Input: part model. Units: mm. Frame: model coordinates. A direction names the side the tool comes from. Round coordinates to 2 decimals unless told otherwise and drop trailing zeros. Order: outer loops, then holes, each group sorted by start corner. A loop starts at its lowest first (then second) coordinate and runs counter-clockwise, first axis right, second up.
Item 1: Cut plane D-D on y = 64. Output: boundary loops of the cut face in (x, z).
Item 2: Reachability of faces 5 (the flat face through (-58, 21, 0)), 6 (the flat face through (-58, 74, 73)), 7 (the flat face through (-58, 67, 58.25)) from +Z, -Z, +X, -X, +Y, -Y: full face, straight path, thin tool, end or side. Return the list, or none.
Item 3: Line query: L1, parallel to Z at x = -57.4, y = 67.25; L2, parallel to Z at x = -57.95, y = -17; L3, parallel to Z at x = -56.8, y = 68.5. Output: solid intervals per line, ascending.
Item 4: Cut plane A-A on y = 13.5. Output: boundary loops of the cut face in (x, z).
Item 5: Mould query, pull axis Y, two halves, no side actions, for faces 1 (the flat face through (-58, -33.5, 5)), 2 (the flat face through (-58, -38.5, 37)), 3 (the flat face through (-58, 22, 6)), 4 (the flat face through (-56.5, 21, 37)). Classes: released by +Y, released by -Y, zero draft, split by the parting line, or undercut.
Item 6: Cut plane B-B on z = 66. Output: boundary loops of the cut face in (x, y).
Item 7: Cut plane C-C on x = -58.75. Output: boundary loops of the cut face in (y, z), then the cut area to 3 significant figures.
Item 8: First-contact query: pin 1 (1.5 mm diameter, centred on x = -58.5, y = 72.5, fed in from +Z). Flat tip, straight axial feed; report the tip coordinate or a pass-through.
Autodesk Inventor part; units mm, degrees
ref_plane "YZ Plane" through (0, 0, 0) normal (1, 0, 0) x (0, 1, 0)
ref_plane "XZ Plane" through (0, 0, 0) normal (0, 1, 0) x (-1, 0, 0)
ref_plane "XY Plane" through (0, 0, 0) normal (0, 0, 1) x (1, 0, 0)
sketch "Sketch1" plane through (0, 0, 0) normal (0, 0, 1) x (1, 0, 0)
  line L0 (-56.5, -25) -> (-59.5, -25)
  line L1 (-59.5, -25) -> (-59.5, 65)
  line L2 (-56.5, -38) -> (-56.5, 78)
  line L3 (-59.5, 65) -> (-56.5, 65)
  line L4 (-56.5, -25) -> (-59.5, -25)
  line L5 (-59.5, -25) -> (-59.5, 65)
  line L6 (-59.5, 65) -> (-56.5, 65)
  line L7 (-56.5, 65) -> (-56.5, -25)
  point P0 (0, 0)
extrude "Extrusion1" add sketch "Sketch1" along normal blind 76
sketch "Sketch2" plane through (-59.5, -25, 0) normal (0, -1, 0) x (1, 0, 0)
  line L0 (3, 0) -> (3, 76)
  line L1 (0, 76) -> (3, 76)
  line L2 (3, 0) -> (0, 0)
  line L3 (0, 0) -> (0, 76)
  line L4 (0, 76) -> (3, 76)
  line L5 (3, 76) -> (3, 0)
  point P0 (59.5, 0)
extrude "Extrusion2" add sketch "Sketch2" along normal blind 13.5
sketch "Sketch4" plane through (-59.5, 65, 0) normal (0, 1, 0) x (1, 0, 0)
  line L0 (3, 0) -> (3, -76)
  line L1 (3, 0) -> (0, 0)
  line L2 (3, -76) -> (0, -76)
  line L3 (0, -76) -> (0, 0)
  line L4 (0, 0) -> (3, 0)
  line L5 (3, 0) -> (3, -76)
  point P0 (59.5, 0)
extrude "Extrusion3" add sketch "Sketch4" along normal blind 16.5
sketch "Sketch5" plane through (-59.5, -38.5, 0) normal (-1, 0, 0) x (0, 0, 1)
  line L0 (0, 120) -> (76, 120)
  line L1 (76, 120) -> (73, 120)
  line L2 (73, 120) -> (73, 110)
  line L3 (73, 110) -> (76, 110)
  line L4 (76, 110) -> (76, 120)
  line L5 (76, 0) -> (76, 120)
  line L6 (76, 0) -> (73, 0)
  line L7 (73, 0) -> (73, 10)
  line L8 (73, 10) -> (76, 10)
  line L9 (76, 10) -> (76, 0)
  point P0 (0, 38.5)
  dimension "d10" = 3
  dimension "d11" = 10
  dimension "d12" = 3
  dimension "d13" = 10
extrude "Extrusion4" cut sketch "Sketch5" against normal blind 10
sketch "Sketch6" plane through (0, 0, 76) normal (0, 0, 1) x (1, 0, 0)
  line L0 (-59.5, -28.5) -> (-56.5, -28.5)
  line L1 (-56.5, -28.5) -> (-56.5, -38.5)
  line L2 (-59.5, -38.5) -> (-59.5, -28.5)
  line L3 (-56.5, -23.5) -> (-59.5, -23.5)
  line L4 (-59.5, 66.5) -> (-56.5, 66.5)
  line L5 (-59.5, 81.5) -> (-59.5, -38.5)
  line L6 (-56.5, -23.5) -> (-59.5, -23.5)
  line L7 (-59.5, -23.5) -> (-59.5, -38.5)
  line L8 (-59.5, -38.5) -> (-56.5, -38.5)
  line L9 (-56.5, -38.5) -> (-56.5, -23.5)
  line L10 (-56.5, 66.5) -> (-59.5, 66.5)
  line L11 (-59.5, 66.5) -> (-59.5, 81.5)
  line L12 (-59.5, 81.5) -> (-56.5, 81.5)
  line L13 (-56.5, 81.5) -> (-56.5, 66.5)
  point P0 (0, 0)
  dimension "d16" = 15
extrude "Extrusion5" cut sketch "Sketch6" against normal blind 3
sketch "Sketch7" plane through (-56.5, -38.5, 0) normal (1, 0, 0) x (0, 0, -1)
  circle A0 centre (-58, 105) radius 5
  circle A1 centre (-58, 105) radius 5
  line L0 (-70, 94.5) -> (-43, 94.5)
  line L1 (-43, 94.5) -> (-43, 117.0005)
  line L2 (-43, 117.0005) -> (-70, 117.0005)
  line L3 (-70, 117.0005) -> (-70, 94.5)
  line L4 (0, 91.5) -> (-73, 91.5)
  line L5 (-73, 105) -> (-73, 95)
  line L6 (-63, 120.0005) -> (-73, 120.0005)
  line L7 (-40, 95) -> (-40, 117)
  line L8 (-58.25, 97.2505) -> (-58.25, 114.2505)
  line L9 (-58.25, 114.2505) -> (-58.25, 97.2505)
  line L10 (-58.25, 97.2505) -> (-67.25, 97.2505)
  line L11 (-67.25, 97.2505) -> (-67.25, 114.2505)
  line L12 (-67.25, 114.2505) -> (-58.25, 114.2505)
  line L13 (-58.25, 114.2505) -> (-67.25, 114.2505)
  line L14 (-67.25, 114.2505) -> (-67.25, 97.2505)
  line L15 (-67.25, 97.2505) -> (-58.25, 97.2505)
  line L16 (-58.25, 97.2505) -> (-58.25, 114.2505)
  circle A2 centre (-49.0313, 105.75) radius 6
  line L17 (-73, 120) -> (0, 120)
  point P0 (0, 38.5)
  point P1 (-58.25, 100.0063)
  point P2 (-58.25, 109.9937)
  dimension "d26" = 3
  dimension "d27" = 3
  dimension "d28" = 3
  dimension "d29" = 3
  dimension "d30" = 12
  dimension "d31" = 9
  dimension "d32" = 14.25
  dimension "d33" = 14.25
extrude "Extrusion6" cut sketch "Sketch7" against normal blind 3 contours A0 A2 | A0 A2 | L8 A0 | A0 L8 L10 L11 L12
sketch "Sketch8" plane through (-59.5, -38.5, 0) normal (-1, 0, 0) x (0, 0, 1)
  line L0 (40, 117) -> (40, 95)
  line L1 (37, 95) -> (37, 117)
  line L2 (37, 117) -> (40, 117)
  line L3 (37, 117) -> (40, 117)
  line L4 (40, 117) -> (40, 95)
  line L5 (40, 95) -> (37, 95)
  line L6 (37, 95) -> (37, 117)
  point P0 (0, 38.5)
  point P1 (37, 95)
extrude "Extrusion7" cut sketch "Sketch8" against normal blind 3
sketch "Sketch9" plane through (-56.5, -38.5, 0) normal (1, 0, 0) x (0, 0, -1)
  line L0 (-6, 115) -> (-6, 5)
  line L1 (-3, 5) -> (-3, 115)
  line L2 (-3, 115) -> (-6, 115)
  line L3 (-6, 5) -> (-3, 5)
  line L4 (-6, 115) -> (-3, 115)
  line L5 (-3, 115) -> (-3, 5)
  line L6 (-3, 5) -> (-6, 5)
  line L7 (-6, 5) -> (-6, 115)
  point P0 (0, 38.5)
extrude "Extrusion8" cut sketch "Sketch9" against normal blind 3
sketch "Sketch10" plane through (-56.5, -38.5, 0) normal (1, 0, 0) x (0, 0, -1)
  point P0 (0, 38.5)
properties part number "divider"
From the geometry:
1. outline: (-59.5, 0) - (-56.5, 0) - (-56.5, 3) - (-59.5, 3) - close; (-59.5, 6) - (-56.5, 6) - (-56.5, 37) - (-59.5, 37) - close; (-59.5, 40) - (-56.5, 40) - (-56.5, 43.99) - (-59.5, 43.99) - close; (-59.5, 54.07) - (-56.5, 54.07) - (-56.5, 58.25) - (-59.5, 58.25) - close; (-59.5, 67.25) - (-56.5, 67.25) - (-56.5, 76) - (-59.5, 76) - close
2. face 5: -Z, +X, -X, +Y, -Y
2. face 6: +Z, +X, -X, +Y
2. face 7: +X, -X
3. L1: z = 0 to 3, 6 to 37, 40 to 43.03, 55.03 to 58.25, 67.25 to 73
3. L2: z = 0 to 3, 6 to 76
3. L3: z = 0 to 3, 6 to 37, 40 to 43.16, 54.9 to 58.25, 67.25 to 73
4. outline: (-59.5, 0) - (-56.5, 0) - (-56.5, 3) - (-59.5, 3) - close; (-59.5, 6) - (-56.5, 6) - (-56.5, 76) - (-59.5, 76) - close
5. face 1: undercut
5. face 2: released by -Y
5. face 3: undercut
5. face 4: zero draft
6. outline: (-59.5, -38.5) - (-56.5, -38.5) - (-56.5, 58.75) - (-59.5, 58.75) - close; (-59.5, 75.75) - (-56.5, 75.75) - (-56.5, 81.5) - (-59.5, 81.5) - close
7. outline: (-38.5, 0) - (81.5, 0) - (81.5, 73) - (66.5, 73) - (66.5, 76) - (-23.5, 76) - (-23.5, 73) - (-38.5, 73) - close; hole (-33.5, 3) - (76.5, 3) - (76.5, 6) - (-33.5, 6) - close; hole (56.5, 37) - (78.5, 37) - (78.5, 40) - (56.5, 40) - close; hole (58.75, 58.25) - (75.75, 58.25) - (75.75, 67.25) - (58.75, 67.25) - close; hole circle Ø12 at (67.25, 49.03)
7. area: 8,370 mm2
8. pin 1: stops at z = 73
